```python
from build123d import *

# Parameters (mm, degrees)
F0_W     = 1.6
F0_H     = 0.8
F0_W_2   = 0.8
F0_H_2   = 0.5
F1_DEPTH = 4
F2_DEPTH = 5


with BuildPart() as f1:
    # F0 (on Top) → F1 (new body)
    with BuildSketch(Plane.XY):
        with Locations((1.2, -0.65)):
            Rectangle(F0_W, F0_H)
        with Locations((0, 0.65)):
            Rectangle(F0_W_2, F0_H)
        with Locations((1.2, 0)):
            Rectangle(F0_W, F0_H_2)
        with Locations((0, -0.65)):
            Rectangle(F0_W_2, F0_H)
        with Locations((-1.2, -0.65)):
            Rectangle(F0_W, F0_H)
        with Locations((-1.2, 0.65)):
            Rectangle(F0_W, F0_H)
        with Locations((1.2, 0.65)):
            Rectangle(F0_W, F0_H)
        with Locations((-1.2, 0)):
            Rectangle(F0_W, F0_H_2)
        Rectangle(F0_W_2, F0_H_2)
    extrude(amount=-F1_DEPTH)

    # F0 (on Top) → F2 (join)
    with BuildSketch(Plane.XY):
        with Locations((1.2, 0.65)):
            Rectangle(F0_W, F0_H)
        with Locations((-1.2, 0.65)):
            Rectangle(F0_W, F0_H)
        with Locations((1.2, -0.65)):
            Rectangle(F0_W, F0_H)
        with Locations((-1.2, -0.65)):
            Rectangle(F0_W, F0_H)
    extrude(amount=F2_DEPTH)

    # F3: F1 across face


with BuildPart() as f1_1:
    add(f1.part)
    add(f1.part.mirror(Plane(origin=(0, -1.05, 0.25), x_dir=(1, 0, 0), z_dir=(0, -1, 0))))

    # F4: F1 across face


with BuildPart() as f1_2:
    add(f1_1.part)
    add(f1_1.part.mirror(Plane(origin=(0, -3.15, 0.25), x_dir=(1, 0, 0), z_dir=(0, -1, 0))))

    # F5: F1 across face


with BuildPart() as f1_3:
    add(f1_2.part)
    add(f1_2.part.mirror(Plane(origin=(0, -7.35, 0.25), x_dir=(1, 0, 0), z_dir=(0, -1, 0))))

    # F6: F1 across face


with BuildPart() as f1_4:
    add(f1_3.part)
    add(f1_3.part.mirror(Plane(origin=(0, -15.75, 0.25), x_dir=(1, 0, 0), z_dir=(0, -1, 0))))

    # F7: F1 across face


with BuildPart() as f1_5:
    add(f1_4.part)
    add(f1_4.part.mirror(Plane(origin=(-2, -15.75, 0.1951219512), x_dir=(0, -1, 0), z_dir=(-1, 0, 0))))


solid = f1_5.part
```
Geometry: final body of the model. Coordinates: model frame, mm. A direction names the side the tool comes from. Round coordinates to 2 decimals unless told otherwise and drop trailing zeros. Order: outer loops, then holes, each group sorted by start corner. A loop starts at its lowest first (then second) coordinate and runs counter-clockwise, first axis right, second up. Notation, with made-up numbers: (47.5, 48.5) -> (95.5, 48.5) arc R32 cw to (95.5, 80.5) -> close; hole circle Ø8 at (15, 83.5). An arc over 180 degrees is marked (long way). Use one line per item in the form item = value.
(1) Section A-A on y = -28. Return loops of the section in (x, z).
Results list:
outline = (-6, -4) -> (2, -4) -> (2, 5) -> (0.4, 5) -> (0.4, 0) -> (-0.4, 0) -> (-0.4, 5) -> (-3.6, 5) -> (-3.6, 0) -> (-4.4, 0) -> (-4.4, 5) -> (-6, 5) -> close
(2) First-contact query: pin 1 Ø1.5 at (x, z) = (0, 3) entering from -Y. Flat tip, straight axial feed; report the tip coordinate or a pass-through.
Results list:
pin_1 = -32.55
(3) Ray query, probe 1 along X at (y, z) = (-2.5, 1.75); probe 2 along Z at (x, y) = (0, -14). Return the intervals inside material, ascending. Write a range as [from, to].
Results list:
probe_1 = [-6, -4.4], [-3.6, -0.4], [0.4, 2]
probe_2 = [-4, 0]
(4) Draft query along Y for faces 4 (the face through (0.4, -14, 2)), 5 (the face through (1, 0.25, 2)). Return one class per face: pulls with the +Y half, pulls with the -Y half, needs draft (parallel to the pull), parting line crosses it, or undercut.
Results list:
face_4 = needs draft
face_5 = undercut
(5) Section B-B on z = 2. Count the separate pieces of the cut face and the enclosed holes in it, and give its area (3 significant figures).
Results list:
separate_pieces = 51
enclosed_holes = 0
area = 164 mm^2
(6) Access query for faces 1 (the face through (-2, -20, 5)), 2 (the face through (-3.6, -14, 2)), 3 (the face through (-2, -1.85, 2)). Directions: +Z, -Z, +X, -X, +Y, -Y. A direction counts if a zero-diameter tool reaches every point of the face in a straight line with its end or side. Return the directions, or none.
Results list:
face_1 = +Z, +X, -X, +Y, -Y
face_2 = +Z, +Y, -Y
face_3 = +Z, +X, -X
